from build123d import *

# Parameters (mm, degrees)
F1_DEPTH = 4.2291
F3_DEPTH = 15.748
F5_DEPTH = 15.748
F7_DEPTH = 15.748


with BuildPart() as f1:
    # F0 (on Right) → F1 (new body, symmetric)
    with BuildSketch(Plane.YZ):
        Polygon((15.748, 0), (-15.748, 0), (-15.748, -1.524), (-9.906, -1.524), (-9.906, -2.54), (-1.016, -2.54), (-1.016, -1.524), (7.874, -1.524), (7.874, -2.54), (15.748, -2.54), align=None)
    extrude(amount=F1_DEPTH, both=True)

    # F2 (on Front) → F3 (join, symmetric)
    with BuildSketch(Plane.XZ):
        with BuildLine():
            Line((-4.2291, -2.54), (-4.2291, 0))
            ThreePointArc((-4.2291, 0), (0, -22.775418), (4.2291, 0))
            Line((4.2291, 0), (4.2291, -2.54))
            ThreePointArc((4.2291, -2.54), (0, -20.448815), (-4.2291, -2.54))
        make_face()
    extrude(amount=F3_DEPTH, both=True)

    # F4 (on Front) → F5 (join, symmetric)
    with BuildSketch(Plane.XZ):
        Polygon((4.21976, 0), (6.25176, 0), (6.25176, 2.54), (-6.27044, 2.53999), (-6.263331, 0), (-4.231331, 0), (-4.231331, 2.024057), (4.21976, 2.024057), align=None)
    extrude(amount=F5_DEPTH, both=True)

    # F6 (on Front) → F7 (join, symmetric)
    with BuildSketch(Plane.XZ):
        with BuildLine():
            ThreePointArc((4.2291, 0), (8.459615, -6.247831), (11.558468, -13.127494))
            ThreePointArc((11.558468, -13.127494), (10.93358, -4.606689), (6.25176, 2.54))
            Line((6.25176, 2.54), (4.2291, 0))
        make_face()
        with BuildLine():
            Line((-4.2291, 0), (-6.27044, 2.53999))
            ThreePointArc((-6.27044, 2.53999), (-10.850879, -4.640597), (-11.567703, -13.127494))
            ThreePointArc((-11.567703, -13.127494), (-8.993183, -5.951736), (-4.2291, 0))
        make_face()
    extrude(amount=F7_DEPTH, both=True)


solid = f1.part
Could you check a few things on this model? Use its own coordinates, in mm. A direction names the side the tool comes from. Coordinates: 2 decimals unless noted, no trailing zeros. Order: outer loops, then holes, each group sorted by start corner. A loop starts at its lowest first (then second) coordinate and runs counter-clockwise, first axis right, second up.
Q1. Will these pins go through, and if not, where does the flat tip stop? pin 1 (0.8 mm diameter, centred on y = 5.5, z = -2, fed in from +X); pin 2 (1 mm diameter, centred on y = -0.5, z = 1.5, fed in from +X); pin 3 (1.6 mm diameter, centred on y = -6, z = 1.5, fed in from -X); pin 4 (3 mm diameter, centred on x = 1, y = -12.5, fed in from -Z).
Q2. Suppose I cut it at B-B on z = -18.75. Please give me the cut outline in (x, y).
Q3. Suppose I cut it at D-D on y = 2.5. Give the number of separate pieces and of enclosed holes in the cut face, and give its area (3 significant figures).
Q4. Suppose I cut it at A-A on x = 0. Please give me the cut outline in (y, z), and give its area (3 significant figures).
Q5. Please list where these lines run through material, in increasing order: L1, parallel to Z at x = 0, y = 8.5; L2, parallel to X at y = -2, z = 0.75; L3, parallel to X at y = 9.5, z = -12.75.
Q6. Thinking about a two-plate mould opening in Z: for faces 4 (the flat face through (0, 0, 2.54)), 5 (the flat face through (0, 12, -2.54)), which applies, released by +Z, released by -Z, zero draft, split by the parting line, or undercut?
Q7. Suppose I cut it at C-C on x = -7.75. Please give me the cut outline in (y, z), and give its area (3 significant figures).
Q8. Which directions (+Z, -Z, +X, -X, +Y, -Y) give clear straight access to the entire face, cutting with the end or side of a thin tool? Please do faces 1 (the flat face through (0, 3, -1.524)), 2 (the flat face through (0, -6, -2.54)), 3 (the flat face through (0, -13, -1.524)).
Answer:
1. pin 1: stops at x = 10.01
1. pin 2: stops at x = 7.75
1. pin 3: stops at x = -7.95
1. pin 4: stops at z = -22.78
2. outline: (-8.87, -15.75) - (-5.41, -15.75) - (-5.41, 15.75) - (-8.87, 15.75) - close; (5.41, -15.75) - (8.87, -15.75) - (8.87, 15.75) - (5.41, 15.75) - close
3. separate pieces: 1
3. enclosed holes: 2
3. area: 193 mm2
4. outline: (-15.75, -22.78) - (15.75, -22.78) - (15.75, -20.45) - (-15.75, -20.45) - close; (-15.75, -1.52) - (-9.91, -1.52) - (-9.91, -2.54) - (-1.02, -2.54) - (-1.02, -1.52) - (7.87, -1.52) - (7.87, -2.54) - (15.75, -2.54) - (15.75, 0) - (-15.75, 0) - close; (-15.75, 2.02) - (15.75, 2.02) - (15.75, 2.54) - (-15.75, 2.54) - close
4. area: 155 mm2
5. L1: z = -22.78 to -20.45, -2.54 to 0, 2.02 to 2.54
5. L2: x = -7.91 to -4.23, 4.22 to 7.96
5. L3: x = -11.65 to -9.29, 9.29 to 11.65
6. face 4: released by +Z
6. face 5: undercut
7. outline: (-15.75, -19.87) - (15.75, -19.87) - (15.75, -16.41) - (-15.75, -16.41) - close; (-15.75, -5.58) - (15.75, -5.58) - (15.75, 0.95) - (-15.75, 0.95) - close
7. area: 315 mm2
8. face 1: none
8. face 2: +Y, -Y
8. face 3: -Y
